Verification items for the finished model (mm, model axes). A direction names the side the tool comes from. Coordinates: 2 decimals unless noted, no trailing zeros. Loops run counter-clockwise (first coordinate to the right, second up) from the corner with the lowest first, then second, coordinate; pieces in that order, holes last. Notation, with made-up numbers: (11, 51.5) - (34, 51.5) arc R20 ccw to (34, 84.5) - close; hole circle Ø8 at (-33, 29.5). An arc over 180 degrees is marked (long way). Answer as CSV lines item,"result". Start each with the question number.
1. Set-up check for faces 1 (the flat face through (30, 0, 2)), 2 (the flat face through (0, 2, 4)), 3 (the flat face through (12, -4, 4)): record each of +Z, -Z, +X, -X, +Y, -Y from which the full face is reachable in a straight line by a thin tool's end or side.
2. Gauge pin test, flat ends, axial feed: P1, Ø2.5, axis at x = 18, y = -3, coming from the -Z side; P2, Ø4, axis at x = 8, z = 6, coming from the -Y side. Record the tip position at first contact, or that the pin passes through.
3. Cross-section at C-C (y = -3). Enter the section's corners in (x, z).
4. Cross-section at B-B (x = 6). Enter the section's corners in (y, z).
5. Material ranges on line 1 (Z direction, x = 6, y = 2.5); line 2 (Y direction, x = 18, z = 5.75); line 3 (X direction, y = 4, z = 2.5), recorded low to high. Write a range as [from, to].
6. Cross-section at D-D (z = 6.5). Enter the section's corners in (x, y).
7. Cross-section at A-A (z = 4). Enter the section's corners in (x, y).
8. Release check for a two-part mould opening along X. For faces 4 (the flat face through (6, 0, 2)), 5 (the flat face through (24, -4, 4)), 6 (the cylindrical face through (5.63, 2.54, 5.66)) record: pulls with the +X half, pulls with the -X half, needs draft (parallel to the pull), parting line crosses it, or undercut.
```python
from build123d import *

# Parameters (mm, degrees)
BOSS_EXTRUDE1_DEPTH  = 8
M3_CLEARANCE_HOLE1_D = 3.4
M3_CLEARANCE_HOLE2_D = 3.4


with BuildPart() as part:
    # Sketch1 → Boss-Extrude1 (new body)
    with BuildSketch(Plane.XY):
        Polygon((0, 0), (0, 5), (36, 5), (36, 0), (24, 0), (24, -8), (12, -8), (12, 0), align=None)
    extrude(amount=BOSS_EXTRUDE1_DEPTH)

    # M3 Clearance Hole1 (through all)
    with Locations(Plane.XY.offset(8)):
        with Locations((18, -3)):
            Hole(M3_CLEARANCE_HOLE1_D / 2)

    # M3 Clearance Hole2 (through all)
    with Locations(Plane(origin=(0, 0, 0), x_dir=(-1, 0, 0), z_dir=(0, -1, 0))):
        with Locations((-6, -4), (-30, -4)):
            Hole(M3_CLEARANCE_HOLE2_D / 2)


solid = part.part
```
Values follow:
1,face 1,"+Z, -Z, +X, -Y"
1,face 2,"+Z, -Z, -X, +Y, -Y"
1,face 3,"+Z, -Z, -X, -Y"
2,P1,"passes through"
2,P2,"stops at y = 0"
3,outline,"(12, 0) - (16.3, 0) - (16.3, 8) - (12, 8) - close; (19.7, 0) - (24, 0) - (24, 8) - (19.7, 8) - close"
4,outline,"(0, 0) - (5, 0) - (5, 2.3) - (0, 2.3) - close; (0, 5.7) - (5, 5.7) - (5, 8) - (0, 8) - close"
5,line 1,"z = [0, 2.3], [5.7, 8]"
5,line 2,"y = [-8, -4.7], [-1.3, 5]"
5,line 3,"x = [0, 5.2], [6.8, 29.2], [30.8, 36]"
6,outline,"(0, 0) - (12, 0) - (12, -8) - (24, -8) - (24, 0) - (36, 0) - (36, 5) - (0, 5) - close; hole circle Ø3.4 at (18, -3)"
7,outline,"(0, 0) - (4.3, 0) - (4.3, 5) - (0, 5) - close; (7.7, 0) - (12, 0) - (12, -8) - (24, -8) - (24, 0) - (28.3, 0) - (28.3, 5) - (7.7, 5) - close; (31.7, 0) - (36, 0) - (36, 5) - (31.7, 5) - close; hole circle Ø3.4 at (18, -3)"
8,face 4,"needs draft"
8,face 5,"pulls with the +X half"
8,face 6,"undercut"
